Build history of the part. All positions in model axes, mm. A direction names the side the tool comes from. Give positions to 0.01 mm unless a question says otherwise; leave off trailing zeros. Loops run counter-clockwise (first coordinate to the right, second up) from the corner with the lowest first, then second, coordinate; pieces in that order, holes last. Notation, with made-up numbers: (3.25, -13.5) -> (20.25, -13.5) arc R30 cw to (20.25, 9.5) -> close; hole circle Ø10 at (9.25, 46). An arc over 180 degrees is marked (long way). Answer as a JSON object with one key per item and string values. Group by question number.
Q1. Tool access for faces 1 (the flat face through (24, 3, 29)), 2 (the flat face through (20, 0, -7)): list every direction of +Z, -Z, +X, -X, +Y, -Y with a clear straight run to the whole face (end or side of a thin tool).
Q2. Drop a flat-ended pin along its axis: pin 1 (4.5 mm diameter, centred on x = 28.5, z = -35, fed in from -Y). Give the stop position or say it passes through.
Q3. Band-saw the part on D-D, the plane z = 17.5. Write the cut outline in (x, y).
Q4. Two-plate mould, pull along X, no slides. Class faces 3 (the cylindrical face through (39.14, 3.04, -46.1)), 4 (the cylindrical face through (34.998, 2.958, 17.247)), 5 (the cylindrical face through (0.86, 3.04, 34.1)), 6 (the cylindrical face through (17.5, 3, 17.6)): pulls with the +X half, pulls with the -X half, needs draft (parallel to the pull), parting line crosses it, or undercut.
Q5. Band-saw the part on B-B, the plane y = 1.3. Write the cut outline in (x, z), plus the area to 3 significant figures.
Q6. Wall check: probe 1 along X at (y, z) = (2, -35); probe 2 along Z at (x, y) = (20, 2.8); probe 3 along X at (y, z) = (4, 5.5). Give the ranges that are in metal, low to high. Write a range as from..to.
Q7. Band-saw the part on A-A, the plane z = -42. Write the cut outline in (x, y), plus the area to 3 significant figures.
Q8. Band-saw the part on C-C, the plane x = 28.5. Write the cut outline in (y, z).
Autodesk Fusion 360 part; units mm, degrees
sketch "Skizze1" plane through (0, 0, 0) normal (0, 1, 0) x (1, 0, 0)
  line L0 (0, 0) -> (40, 0)
  line L1 (40, 0) -> (40, 47)
  line L2 (40, 47) -> (0, 47)
  line L3 (0, 47) -> (0, 0)
  circle A0 centre (20, 42) radius 2.5
  circle A1 centre (28.5, 35) radius 2.5
  circle A2 centre (11.5, 35) radius 2.5
  line L4 (0, 0) -> (40, 0)
  line L5 (40, 0) -> (40, -35)
  line L6 (40, -35) -> (0, -35)
  line L7 (0, -35) -> (0, 0)
  circle A3 centre (20, -17.5) radius 15
  circle A4 centre (20, -17.5) radius 10
  line L8 (16, -3.0432) -> (16, -8.3348)
  line L9 (24, -3.0432) -> (24, -8.3348)
  line L10 (16, -26.6652) -> (16, -31.9568)
  line L11 (24, -26.6652) -> (24, -31.9568)
  circle A5 centre (20, -17.5) radius 2.5
  dimension "d1" = 40
  dimension "d2" = 47
  dimension "d3" = 5
  dimension "d4" = 5
  dimension "d5" = 5
  dimension "d6" = 5
  dimension "d7" = 20
  dimension "d8" = 17
  dimension "d9" = 11.5
  dimension "d11" = 7
  dimension "d12" = 30
  dimension "d13" = 20
  dimension "d14" = 17.5
  dimension "d15" = 35
  dimension "d16" = 8
  dimension "d17" = 4
  dimension "d18" = 8
  dimension "d19" = 4
  dimension "d28" = 5
extrude "Extrusion1" add sketch "Skizze1" along normal blind 6 contours L0 L1 L2 L3 L4 | L0 L4 L5 L6 L7 | A3 A4 L8 L9 | A3 A4 L10 L11 | A4
fillet "Abrundung1" radius 1 4 edges at (24, 3, 3.0432) (24, 3, 26.6652) (24, 3, 8.3348) (24, 3, 31.9568)
fillet "Abrundung1" radius 1 4 edges at (16, 3, 31.9568) (16, 3, 8.3348) (16, 3, 26.6652) (16, 3, 3.0432)
fillet "Abrundung1" radius 3 4 edges at (0, 3, 35) (40, 3, 35) (40, 3, -47) (0, 3, -47)
sketch "Skizze2" plane through (0, 6, 0) normal (0, 1, 0) x (-1, 0, 0)
  arc A0 (-3, -47) -> (0, -44) centre (-3, -44) ccw
  line L0 (0, -44) -> (0, 32)
  arc A1 (0, 32) -> (-3, 35) centre (-3, 32) ccw
  line L1 (-3, 35) -> (-37, 35)
  arc A2 (-37, 35) -> (-40, 32) centre (-37, 32) ccw
  line L2 (-40, 32) -> (-40, -44)
  arc A3 (-40, -44) -> (-37, -47) centre (-37, -44) ccw
  line L3 (-37, -47) -> (-3, -47)
  circle A4 centre (-11.5, -35) radius 2.5
  circle A5 centre (-28.5, -35) radius 2.5
  circle A6 centre (-20, 17.5) radius 2.5
  arc A7 (-14.6429, 3.4893) -> (-14.6429, 31.5107) centre (-20, 17.5) ccw
  arc A8 (-16, 4.4233) -> (-14.6429, 3.4893) centre (-15, 4.4233) ccw
  line L4 (-16, 4.4233) -> (-16, 7.702)
  arc A9 (-15.4545, 8.5928) -> (-16, 7.702) centre (-15, 7.702) ccw
  arc A10 (-15.4545, 8.5928) -> (-15.4545, 26.4072) centre (-20, 17.5) ccw
  arc A11 (-16, 27.298) -> (-15.4545, 26.4072) centre (-15, 27.298) ccw
  line L5 (-16, 27.298) -> (-16, 30.5767)
  arc A12 (-14.6429, 31.5107) -> (-16, 30.5767) centre (-15, 30.5767) ccw
  circle A13 centre (-20, -42) radius 2.5
  line L6 (-24, 30.5767) -> (-24, 27.298)
  arc A14 (-24.5455, 26.4072) -> (-24, 27.298) centre (-25, 27.298) ccw
  arc A15 (-24.5455, 26.4072) -> (-24.5455, 8.5928) centre (-20, 17.5) ccw
  arc A16 (-24, 7.702) -> (-24.5455, 8.5928) centre (-25, 7.702) ccw
  line L7 (-24, 7.702) -> (-24, 4.4233)
  arc A17 (-25.3571, 3.4893) -> (-24, 4.4233) centre (-25, 4.4233) ccw
  arc A18 (-25.3571, 31.5107) -> (-25.3571, 3.4893) centre (-20, 17.5) ccw
  arc A19 (-24, 30.5767) -> (-25.3571, 31.5107) centre (-25, 30.5767) ccw
Worked answers:
{
 "1": {"face 1": "+Y, -Y", "face 2": "+Z, -Z, +X, -X, -Y"},
 "2": {"pin 1": "through"},
 "3": {"outline": "(0, 0) -> (5, 0) -> (5, 6) -> (0, 6) -> close; (10, 0) -> (17.5, 0) -> (17.5, 6) -> (10, 6) -> close; (22.5, 0) -> (30, 0) -> (30, 6) -> (22.5, 6) -> close; (35, 0) -> (40, 0) -> (40, 6) -> (35, 6) -> close"},
 "4": {"face 3": "pulls with the +X half", "face 4": "undercut", "face 5": "pulls with the -X half", "face 6": "undercut"},
 "5": {"outline": "(0, -44) arc R3 ccw to (3, -47) -> (37, -47) arc R3 ccw to (40, -44) -> (40, 32) arc R3 ccw to (37, 35) -> (3, 35) arc R3 ccw to (0, 32) -> close; hole circle Ø5 at (11.5, -35); hole (14.64, 3.49) arc R1 ccw to (16, 4.42) -> (16, 7.7) arc R1 ccw to (15.45, 8.59) arc R10 cw to (15.45, 26.41) arc R1 ccw to (16, 27.3) -> (16, 30.58) arc R1 ccw to (14.64, 31.51) arc R15 ccw to start; hole circle Ø5 at (20, -42); hole circle Ø5 at (20, 17.5); hole (24, 4.42) arc R1 ccw to (25.36, 3.49) arc R15 ccw to (25.36, 31.51) arc R1 ccw to (24, 30.58) -> (24, 27.3) arc R1 ccw to (24.55, 26.41) arc R10 cw to (24.55, 8.59) arc R1 ccw to (24, 7.7) -> close; hole circle Ø5 at (28.5, -35)", "area": "2,880 mm2"},
 "6": {"probe 1": "0..9, 14..26, 31..40", "probe 2": "-47..-44.5, -39.5..15, 20..35", "probe 3": "0..11, 16..24, 29..40"},
 "7": {"outline": "(0, 0) -> (17.5, 0) -> (17.5, 6) -> (0, 6) -> close; (22.5, 0) -> (40, 0) -> (40, 6) -> (22.5, 6) -> close", "area": "210 mm2"},
 "8": {"outline": "(0, -47) -> (6, -47) -> (6, -37.5) -> (0, -37.5) -> close; (0, -32.5) -> (6, -32.5) -> (6, 5.14) -> (0, 5.14) -> close; (0, 12.23) -> (6, 12.23) -> (6, 22.77) -> (0, 22.77) -> close; (0, 29.86) -> (6, 29.86) -> (6, 35) -> (0, 35) -> close"}
}
